CAD build for the part. Positions are in the model's coordinates, mm. A direction names the side the tool comes from. Give positions to 0.01 mm unless a question says otherwise; leave off trailing zeros. Write each loop counter-clockwise with the first axis right and the second up, starting at its lowest first coordinate (ties: lowest second). Pieces come first, ordered by that corner, then holes. Notation, with made-up numbers: (-29, 14) - (17, 14) arc R17 ccw to (17, 44) - close; hole circle Ø6 at (32.5, 49.5). An arc over 180 degrees is marked (long way). Put each result on its own line as item: value. Start each with the question number.
1. Cut at A-A on x = 32. List the corners of the cut face in (y, z), and give its area (3 significant figures).
2. Mould opens along Y. For faces 1 (the cylindrical face through (31.272, -119.276, -0.986)), 2 (the cylindrical face through (-7.32, -190.75, 136.57)), 3 (the flat face through (18, -91, 0)), 4 (the cylindrical face through (29.451, -20.223, -0.986)) say: +Y half, -Y half, draft (parallel to the pull), parting line (faces both ways), or undercut.
3. Wall check: line 1 (X direction, y = -106.5, z = 106.5); line 2 (Z direction, x = -4, y = -151). Give the ranges that are in metal, low to high.
4. Drop flat-ended pins along their axis: pin 1 (10 mm diameter, centred on x = 28, y = -157.5, fed in from +Z); pin 2 (4 mm diameter, centred on y = -59, z = 103.5, fed in from +X). Give the stop position or say it passes through.
5. Cut at B-B on y = -61.5. List the corners of the cut face in (x, z), and give its area (3 significant figures).
6. Cut at D-D on z = 109. List the corners of the cut face in (x, y), and give its area (3 significant figures).
7. Cut at C-C on x = 10.5. List the corners of the cut face in (y, z), and give its area (3 significant figures).
8. Tool access for faces 5 (the flat face through (-6.338, -91, 70)), 6 (the flat face through (18, -91, -2)): list every direction of +Z, -Z, +X, -X, +Y, -Y with a clear straight run to the whole face (end or side of a thin tool).
from build123d import *

# Parameters (mm, degrees)
SKETCH_1_W                       = 50
SKETCH_1_H                       = 200
SM_BASE_FLANGE_1_DEPTH           = 2
SM_EDGE_FLANGE_1_STRIP_W         = 9.4732
SM_EDGE_FLANGE_1_STRIP_H         = 2
SM_EDGE_FLANGE_1_STRIP_CUT_DEPTH = 200
SM_EDGE_FLANGE_1_DEPTH           = 200
SKETCH_8_R                       = 3
CUT_EXTRUDE_1_DEPTH              = 10
PATTERN_LINEAR_1_COUNT           = 2
PATTERN_LINEAR_1_PITCH           = 100
FILLET_2_R                       = 5
FILLET_3_R                       = 5


# Sheet-metal steps are written as plain solids
with BuildPart() as part:
    # Sketch 1 → 基体-法兰1 (new body)
    with BuildSketch(Plane.XY):
        with Locations((16.662404092, -92.250639386)):
            Rectangle(SKETCH_1_W, SKETCH_1_H)
    extrude(amount=-SM_BASE_FLANGE_1_DEPTH)

    # 边线-法兰1 strip (across the edge) → 边线-法兰1 strip cut (cut)
    with BuildSketch(Plane(origin=(-8.337595908, 7.749360614, 0), x_dir=(1, 0, 0), z_dir=(0, -1, 0))):
        with Locations((-2, -1)):
            Rectangle(SM_EDGE_FLANGE_1_STRIP_W, SM_EDGE_FLANGE_1_STRIP_H)
    extrude(amount=SM_EDGE_FLANGE_1_STRIP_CUT_DEPTH, mode=Mode.SUBTRACT)

    # 边线-法兰1 section (across the edge) → 边线-法兰1 (add)
    with BuildSketch(Plane(origin=(-8.337595908, 7.749360614, 0), x_dir=(1, 0, 0), z_dir=(0, -1, 0))):
        with BuildLine():
            Line((0, 0.7366), (0, 138))
            Line((0, 138), (2, 138))
            Line((2, 138), (2, 0.7366))
            ThreePointArc((2, 0.7366), (2.215745145, 0.215745145), (2.7366, 0))
            Line((2.7366, 0), (2.7366, -2))
            ThreePointArc((2.7366, -2), (0.801531583, -1.198468417), (0, 0.7366))
        make_face()
    extrude(amount=SM_EDGE_FLANGE_1_DEPTH)

    # 草图8 → 切除-拉伸1 (cut)
    with BuildSketch(Plane.XY):
        with Locations((31.662404092, -22.250639386)):
            Circle(SKETCH_8_R)
    cut_extrude_1 = extrude(amount=-CUT_EXTRUDE_1_DEPTH, mode=Mode.SUBTRACT)

    # 阵列(线性)1: 切除-拉伸1 ×2
    with Locations(*[(0, -i * PATTERN_LINEAR_1_PITCH, 0) for i in range(1, PATTERN_LINEAR_1_COUNT)]):
        add(cut_extrude_1, mode=Mode.SUBTRACT)

    # 圆角2
    fillet_2_edges = [part.edges().sort_by_distance(p)[0] for p in [
        (-7.337595908, 7.749360614, 138),
    ]]
    fillet(fillet_2_edges, radius=FILLET_2_R)

    # 圆角3
    fillet_3_edges = [part.edges().sort_by_distance(p)[0] for p in [
        (-7.337595908, -192.250639386, 138),
    ]]
    fillet(fillet_3_edges, radius=FILLET_3_R)


solid = part.part
Report:
1. outline: (-192.25, -2) - (-125.23, -2) - (-125.23, 0) - (-192.25, 0) - close; (-119.27, -2) - (-25.23, -2) - (-25.23, 0) - (-119.27, 0) - close; (-19.27, -2) - (7.75, -2) - (7.75, 0) - (-19.27, 0) - close
1. area: 376 mm²
2. face 1: undercut
2. face 2: -Y half
2. face 3: draft
2. face 4: undercut
3. line 1: x = -8.34 to -6.34
3. line 2: z = -2 to 0
4. pin 1: stops at z = 0
4. pin 2: stops at x = -6.34
5. outline: (-8.34, 0.74) arc R2.74 ccw to (-5.6, -2) - (41.66, -2) - (41.66, 0) - (-5.6, 0) arc R0.74 cw to (-6.34, 0.74) - (-6.34, 138) - (-8.34, 138) - close
5. area: 375 mm²
6. outline: (-8.34, -192.25) - (-6.34, -192.25) - (-6.34, 7.75) - (-8.34, 7.75) - close
6. area: 400 mm²
7. outline: (-192.25, -2) - (7.75, -2) - (7.75, 0) - (-192.25, 0) - close
7. area: 400 mm²
8. face 5: +Z, +X, +Y, -Y
8. face 6: -Z, +X, -X, +Y, -Y
